Work out the finished part from the listing and answer in its coordinate system (mm). Face numbers are marked on the shaded views. Coordinates: 2 decimals unless noted, no trailing zeros. Order: outer loops, then holes, each group sorted by start corner. A loop starts at its lowest first (then second) coordinate and runs counter-clockwise, first axis right, second up. Notation, with made-up numbers: (-38, -36) -> (7, -36) arc R23 cw to (7, -3) -> close; hole circle Ø2 at (-9.75, -22). An arc over 180 degrees is marked (long way). Answer as CSV lines item,"result". Start each with the question number.
Item 1: Section B-B (z = 26) is taken. Write down the section's boundary in (x, y).
Item 2: Straight lines are drawn through the part: L1, parallel to Y at x = 0, z = 4; L2, parallel to Y at x = -9, z = 2; L3, parallel to Y at x = 9, z = 2. For each, find the intervals that lie inside material, in ascending order.
Item 3: Each of these flat-tipped pins is pushed along its axis until it touches: pin 1 Ø5 at (y, z) = (0, 27.5) entering from -X; pin 2 Ø1.7 at (x, y) = (0, -8) entering from +Z; pin 3 Ø8 at (y, z) = (8, 11.5) entering from +X. Where does it stop, or does it pass through?
Item 4: Section A-A (z = 9.5) is taken. Write down the section's boundary in (x, y).
Item 5: For a pull along X with two mould halves and no side action, classify the marked faces 1, 2 and 3 as pulls with the +X half, pulls with the -X half, needs draft (parallel to the pull), parting line crosses it, or undercut.
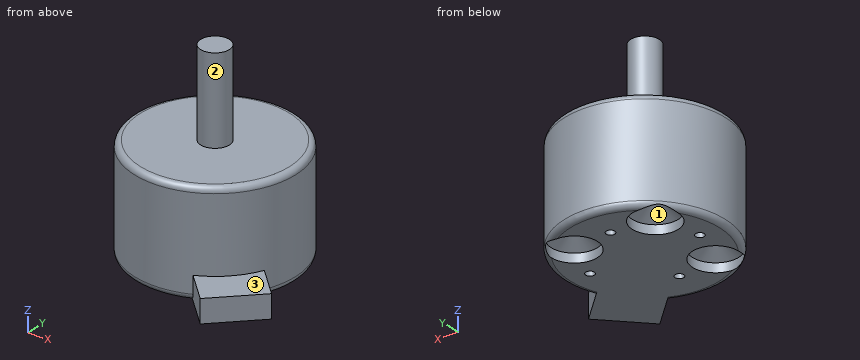
```python
from build123d import *

# Parameters (mm, degrees)
F3_D      = 1.5
F3_DEPTH  = 8
F3_TIP    = 0.4506454643
F7_W      = 9
F7_H      = 4
F8_DEPTH  = 5
F10_D     = 8
F10_DEPTH = 1
F10_START = 0.5630689
F10_TIP   = 2.4034424761


with BuildPart() as f1:
    # F0 (on Front) → F1 (revolve)
    with BuildSketch(Plane.XZ):
        with BuildLine():
            Line((0, 33), (0, 0))
            Line((0, 0), (13, 0))
            ThreePointArc((13, 0), (13.7071067812, 0.2928932188), (14, 1))
            Line((14, 1), (14, 17))
            ThreePointArc((14, 17), (13.7071067812, 17.7071067812), (13, 18))
            Line((13, 18), (2.5, 18))
            Line((2.5, 18), (2.5, 33))
            Line((2.5, 33), (0, 33))
        make_face()
    revolve(axis=Axis((0, 0, 16.5), (0, 0, -1)))

    # F3
    with Locations(Plane(origin=(0, 0, 0), x_dir=(1, 0, 0), z_dir=(0, 0, -1))):
        with Locations((0, 8), (-9.5, 0), (0, -8), (9.5, 0)):
            Hole(F3_D / 2, depth=F3_DEPTH)
            with Locations((0, 0, -(F3_DEPTH + F3_TIP / 2))):  # 118° drill point
                Cone(0, F3_D / 2, F3_TIP, mode=Mode.SUBTRACT)

    # F7 (on 3pt) → F8 (join, symmetric)
    with BuildSketch(Plane(origin=(0, 0, 0), x_dir=(-0.7071067812, 0.7071067812, 0), z_dir=(0.7071067812, 0.7071067812, 0))):
        with Locations((-15.5, 2)):
            Rectangle(F7_W, F7_H)
    extrude(amount=F8_DEPTH, both=True)

    # F10
    # its depths count from where the whole tool has entered the part; down to there all is cleared
    with Locations(Plane(origin=(0, 0, 0), x_dir=(1, 0, 0), z_dir=(0, 0, -1)).offset(-F10_START)):
        with Locations((-7, 7), (-7, -7), (7, -7)):
            Hole(F10_D / 2, depth=F10_DEPTH)
            with Locations((0, 0, -(F10_DEPTH + F10_TIP / 2))):  # 118° drill point
                Cone(0, F10_D / 2, F10_TIP, mode=Mode.SUBTRACT)


solid = f1.part
```
Checked values:
1,outline,"circle Ø5 at (0, 0)"
2,L1,"y = -14 to -8.75, -7.25 to 7.25, 8.75 to 14"
2,L2,"y = -10.72 to -9.59, -4.41 to -0.56, 0.56 to 4.41, 9.59 to 10.72"
2,L3,"y = -16.07 to -0.56, 0.56 to 4.41, 9.59 to 10.72"
3,pin 1,"stops at x = -2.5"
3,pin 2,"stops at z = 18"
3,pin 3,"stops at x = 13.42"
4,outline,"circle Ø28 at (0, 0)"
5,face 1,"undercut"
5,face 2,"parting line crosses it"
5,face 3,"needs draft"
